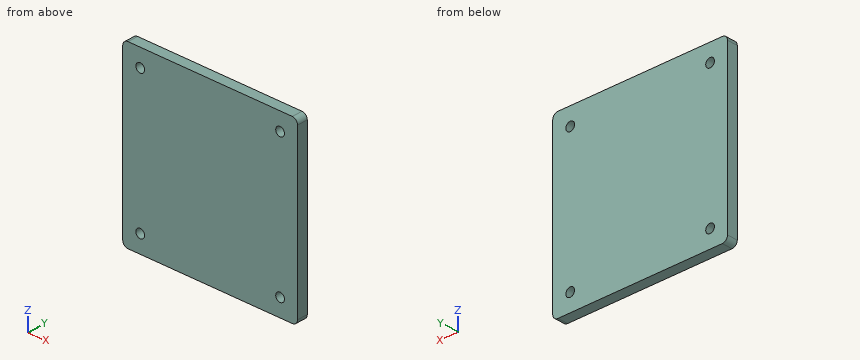
```python
from build123d import *

# Parameters (mm, degrees)
SKETCH1_W           = 100
SKETCH1_H           = 100
SKETCH1_R           = 2.5
BOSS_EXTRUDE1_DEPTH = 6
FILLET1_R           = 3
SCALE1_SCALE        = 7.5


with BuildPart() as part:
    # Sketch1 → Boss-Extrude1 (new body)
    with BuildSketch(Plane(origin=(0, 0, 0), x_dir=(1, 0, 0), z_dir=(0, 1, 0))):
        with Locations((40, -40)):
            Rectangle(SKETCH1_W, SKETCH1_H)
        Circle(SKETCH1_R, mode=Mode.SUBTRACT)
        with Locations((80, 0)):
            Circle(SKETCH1_R, mode=Mode.SUBTRACT)
        with Locations((80, -80)):
            Circle(SKETCH1_R, mode=Mode.SUBTRACT)
        with Locations((0, -80)):
            Circle(SKETCH1_R, mode=Mode.SUBTRACT)
    extrude(amount=BOSS_EXTRUDE1_DEPTH)

    # Fillet1
    fillet1_edges = [part.edges().sort_by_distance(p)[0] for p in [
        (-10, 3, -10),
        (90, 3, -10),
        (90, 3, 90),
        (-10, 3, 90),
    ]]
    fillet(fillet1_edges, radius=FILLET1_R)


with BuildPart() as part_1:
    # Scale1: scaled about (40, 3, 40)
    add(part.part.scale(SCALE1_SCALE).moved(Location((-260, -19.5, -260))))


solid = part_1.part
```
Could you check a few things on this model? Use its own coordinates, in mm. Round coordinates to 2 decimals unless told otherwise and drop trailing zeros. Loops run counter-clockwise (first coordinate to the right, second up) from the corner with the lowest first, then second, coordinate; pieces in that order, holes last. Notation, with made-up numbers: (58, 45.5) -> (111, 45.5) arc R24 ccw to (111, 57.5) -> close; hole circle Ø2 at (59.5, 43.25). An arc over 180 degrees is marked (long way). Put each result on its own line as item: value.
Q1. I want a section at A-A on z = 340. Write out the boundary of the cut face in (x, y).
Checks:
outline: (-335, -19.5) -> (-278.75, -19.5) -> (-278.75, 25.5) -> (-335, 25.5) -> close; (-241.25, -19.5) -> (321.25, -19.5) -> (321.25, 25.5) -> (-241.25, 25.5) -> close; (358.75, -19.5) -> (415, -19.5) -> (415, 25.5) -> (358.75, 25.5) -> close
Q2. I want a section at B-B on x = -260. Write out the boundary of the cut face in (y, z).
Checks:
outline: (-19.5, -335) -> (25.5, -335) -> (25.5, -278.75) -> (-19.5, -278.75) -> close; (-19.5, -241.25) -> (25.5, -241.25) -> (25.5, 321.25) -> (-19.5, 321.25) -> close; (-19.5, 358.75) -> (25.5, 358.75) -> (25.5, 415) -> (-19.5, 415) -> close
Q3. For pin 1 Ø22.5 at (x, z) = (-260, -260) entering from +Y, with a flat end and sliding along its axis, tell me the tip position at first contact or that it passes through.
Checks:
pin 1: through
Q4. Please list where these lines run through material, in increasing order: line 1 (X direction, y = -7, z = -260); line 2 (Z direction, x = 334.5, y = 12.5). Write a range as from..to.
Checks:
line 1: -335..-278.75, -241.25..321.25, 358.75..415
line 2: -335..-277.93, -242.07..322.07, 357.93..415
